Read the model definition and answer for the solid it produces. Units are mm, in the model's axes. A direction names the side the tool comes from. Coordinates: 2 decimals unless noted, no trailing zeros. Loops run counter-clockwise (first coordinate to the right, second up) from the corner with the lowest first, then second, coordinate; pieces in that order, holes last. Notation, with made-up numbers: (33.5, 34) -> (52.5, 34) arc R30 cw to (52.5, 58) -> close; hole circle Ø5 at (47, 52.5). An arc over 180 degrees is marked (long way). Answer in a Markdown table with one row per item.
```python
from build123d import *

# Parameters (mm, degrees)
SKETCH_1_W          = 40
SKETCH_1_H          = 40
EXTRUDE_1_DEPTH     = 3
SKETCH_2_R          = 2
EXTRUDE_2_DEPTH     = 2
SKETCH_3_R          = 0.9
EXTRUDE_3_DEPTH     = 4.15
SKETCH_4_R          = 4
EXTRUDE_4_DEPTH     = 6.15
SKETCH_5_R          = 2.1
CUT_EXTRUDE_1_DEPTH = 10.15


with BuildPart() as part:
    # 草圖1 → 填料-伸長1 (new body)
    with BuildSketch(Plane.XY):
        Rectangle(SKETCH_1_W, SKETCH_1_H)
    extrude(amount=EXTRUDE_1_DEPTH)

    # 草圖2 → 填料-伸長2 (add)
    with BuildSketch(Plane.XY.offset(3)):
        with Locations((-7.62, 10.795)):
            Circle(SKETCH_2_R)
        with Locations((-7.62, -10.795)):
            Circle(SKETCH_2_R)
        with Locations((7.62, 10.795)):
            Circle(SKETCH_2_R)
        with Locations((7.62, -10.795)):
            Circle(SKETCH_2_R)
    extrude(amount=EXTRUDE_2_DEPTH)

    # 草圖3 → 填料-伸長3 (add)
    with BuildSketch(Plane.XY.offset(5)):
        with Locations((-7.62, 10.795)):
            Circle(SKETCH_3_R)
        with Locations((-7.62, -10.795)):
            Circle(SKETCH_3_R)
        with Locations((7.62, -10.795)):
            Circle(SKETCH_3_R)
        with Locations((7.62, 10.795)):
            Circle(SKETCH_3_R)
    extrude(amount=EXTRUDE_3_DEPTH)

    # 草圖4 → 填料-伸長4 (add)
    with BuildSketch(Plane.XY.offset(3)):
        with Locations((-15, 15)):
            Circle(SKETCH_4_R)
        with Locations((-15, -15)):
            Circle(SKETCH_4_R)
        with Locations((15, -15)):
            Circle(SKETCH_4_R)
        with Locations((15, 15)):
            Circle(SKETCH_4_R)
    extrude(amount=EXTRUDE_4_DEPTH)

    # 草圖5 → 除料-伸長1 (cut, through all)
    with BuildSketch(Plane.XY.offset(9.15)):
        with Locations((-15, 15)):
            Circle(SKETCH_5_R)
        with Locations((-15, -15)):
            Circle(SKETCH_5_R)
        with Locations((15, -15)):
            Circle(SKETCH_5_R)
        with Locations((15, 15)):
            Circle(SKETCH_5_R)
    extrude(amount=-CUT_EXTRUDE_1_DEPTH, mode=Mode.SUBTRACT)


solid = part.part
```
1. A tool of negligible diameter and unlimited length cuts with its end or side. For faces 4 (the cylindrical face through (-15.273, -12.918, 4.639)), 5 (the flat face through (8, -12, 5)), from which of +Z, -Z, +X, -X, +Y, -Y can it reach the whole face along a straight path? Write none if from no direction.
A:
| item | result |
|---|---|
| face 4 | +Z, -Z |
| face 5 | +Z |
2. Find the intervals of material crossed by probe 1 along Y at (x, z) = (15, 4.5); probe 2 along Y at (x, z) = (-15, 2.5); probe 3 along X at (y, z) = (-14, 7), in increasing order.
A:
| item | result |
|---|---|
| probe 1 | y = -19 to -17.1, -12.9 to -11, 11 to 12.9, 17.1 to 19 |
| probe 2 | y = -20 to -17.1, -12.9 to 12.9, 17.1 to 20 |
| probe 3 | x = -18.87 to -16.85, -13.15 to -11.13, 11.13 to 13.15, 16.85 to 18.87 |
3. A cutting plane is placed at C-C on z = 8.5. Count the separate pieces of the cut face and the enclosed holes in it, and give its area (3 significant figures).
A:
| item | result |
|---|---|
| separate pieces | 8 |
| enclosed holes | 4 |
| area | 156 mm2 |
4. A cutting plane is placed at D-D on x = 7.62. Give the vertices of the cut face in (y, z) (3 decimals).
A:
| item | result |
|---|---|
| outline | (-20, 0) -> (20, 0) -> (20, 3) -> (12.795, 3) -> (12.795, 5) -> (11.695, 5) -> (11.695, 9.15) -> (9.895, 9.15) -> (9.895, 5) -> (8.795, 5) -> (8.795, 3) -> (-8.795, 3) -> (-8.795, 5) -> (-9.895, 5) -> (-9.895, 9.15) -> (-11.695, 9.15) -> (-11.695, 5) -> (-12.795, 5) -> (-12.795, 3) -> (-20, 3) -> close |
5. The mould has two halves that part along X. Classify faces 1 (the cylindrical face through (14.727, -12.918, 4.639)), 2 (the flat face through (-8, -11, 9.15)), 3 (the flat face through (-20, 0, 1)): pulls with the +X half, pulls with the -X half, needs draft (parallel to the pull), parting line crosses it, or undercut.
A:
| item | result |
|---|---|
| face 1 | undercut |
| face 2 | needs draft |
| face 3 | pulls with the -X half |
6. A cutting plane is placed at A-A on y = -15. Give the vertices of the cut face in (x, z), and give its area (3 significant figures).
A:
| item | result |
|---|---|
| outline | (-20, 0) -> (-17.1, 0) -> (-17.1, 9.15) -> (-19, 9.15) -> (-19, 3) -> (-20, 3) -> close; (-12.9, 0) -> (12.9, 0) -> (12.9, 9.15) -> (11, 9.15) -> (11, 3) -> (-11, 3) -> (-11, 9.15) -> (-12.9, 9.15) -> close; (17.1, 0) -> (20, 0) -> (20, 3) -> (19, 3) -> (19, 9.15) -> (17.1, 9.15) -> close |
| area | 142 mm2 |
7. Given pin 1 Ø1.5 at (x, y) = (1.5, 5.5) entering from +Z, flat-ended and moving along its own axis, determine where the tip first touches the part or whether it passes through.
A:
| item | result |
|---|---|
| pin 1 | stops at z = 3 |
